Verification items for the finished model (mm, model axes). Give positions to 0.01 mm unless a question says otherwise; leave off trailing zeros. Write each loop counter-clockwise with the first axis right and the second up, starting at its lowest first coordinate (ties: lowest second). Pieces come first, ordered by that corner, then holes.
from build123d import *

# Parameters (mm, degrees)
F1_DEPTH = 3.5
F2_R     = 1.8
F3_DEPTH = 6
F4_R     = 1.8
F5_DEPTH = 6


with BuildPart() as f1:
    # F0 (on Top) → F1 (new body, symmetric)
    with BuildSketch(Plane.XY):
        with BuildLine():
            ThreePointArc((45, 1), (40.899495, 10.899495), (31, 15))
            Line((31, 15), (-31, 15))
            ThreePointArc((-31, 15), (-40.899495, 10.899495), (-45, 1))
            Line((-45, 1), (-45, -1))
            ThreePointArc((-45, -1), (-40.899495, -10.899495), (-31, -15))
            Line((-31, -15), (31, -15))
            ThreePointArc((31, -15), (40.899495, -10.899495), (45, -1))
            Line((45, -1), (45, 1))
        make_face()
    extrude(amount=F1_DEPTH, both=True)

    # F2 (on face) → F3 (cut)
    with BuildSketch(Plane.XY.offset(3.5)):
        with Locations((39.474629, 0)):
            Circle(F2_R)
    extrude(amount=-F3_DEPTH, mode=Mode.SUBTRACT)

    # F4 (on face) → F5 (cut)
    with BuildSketch(Plane.XY.offset(3.5)):
        with Locations((-41.609546, 0)):
            Circle(F4_R)
    extrude(amount=-F5_DEPTH, mode=Mode.SUBTRACT)


solid = f1.part
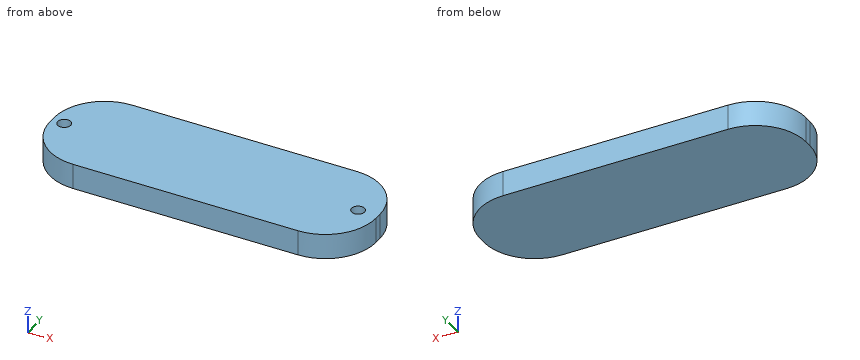
Item 1: Sectioned sample at B-B on y = 0. Record the cut outline in (x, z).
Answer key:
outline: (-45, -3.5) - (45, -3.5) - (45, 3.5) - (41.27, 3.5) - (41.27, -2.5) - (37.67, -2.5) - (37.67, 3.5) - (-39.81, 3.5) - (-39.81, -2.5) - (-43.41, -2.5) - (-43.41, 3.5) - (-45, 3.5) - close
Item 2: Sectioned sample at D-D on y = 10. Record the cut outline in (x, z).
Answer key:
outline: (-41.72, -3.5) - (41.72, -3.5) - (41.72, 3.5) - (-41.72, 3.5) - close
Item 3: Scan lines: line 1 along X through (y, z) = (0.5, -2.25); line 2 along X through (y, z) = (-8, 0.5); line 3 along Y through (x, z) = (35, -2.75). Record each from-to range of solid material in increasing order.
Answer key:
line 1: x = -45 to -43.34, -39.88 to 37.75, 41.2 to 45
line 2: x = -43.12 to 43.12
line 3: y = -14.42 to 14.42
Item 4: Sectioned sample at C-C on x = 34. Record the cut outline in (y, z).
Answer key:
outline: (-14.67, -3.5) - (14.67, -3.5) - (14.67, 3.5) - (-14.67, 3.5) - close
Item 5: Sectioned sample at A-A on z = 0.5. Record the cut outline in (x, y).
Answer key:
outline: (-45, -1) arc R14 ccw to (-31, -15) - (31, -15) arc R14 ccw to (45, -1) - (45, 1) arc R14 ccw to (31, 15) - (-31, 15) arc R14 ccw to (-45, 1) - close; hole circle Ø3.6 at (-41.61, 0); hole circle Ø3.6 at (39.47, 0)
Item 6: Depth check by flat-ended pin: pin 1 (4 mm diameter, centred on y = -5, z = 1.5, fed in from -X); pin 2 (1.1 mm diameter, centred on x = -42, y = 0.5, fed in from +Z); pin 3 (2 mm diameter, centred on y = 9, z = 1, fed in from +X). Enter the tip coordinate at first touch or a pass-through.
Answer key:
pin 1: stops at x = -44.86
pin 2: stops at z = -2.5
pin 3: stops at x = 43.12
